Geometry: final body of the model. Coordinates: model frame, mm. A direction names the side the tool comes from. Give positions to 0.01 mm unless a question says otherwise; leave off trailing zeros. Write each loop counter-clockwise with the first axis right and the second up, starting at its lowest first coordinate (ties: lowest second). Pieces come first, ordered by that corner, then holes.
```python
from build123d import *

# Parameters (mm, degrees)
F0_W          = 19
F0_H          = 19
F3_DEPTH      = 2
F4_START      = 2
F2_W          = 19
F2_H          = 14
F4_DEPTH      = 9.5
F5_START      = 11.5
F1_R          = 6
F5_DEPTH      = 7.5
F6_R          = 1
F7_DEPTH      = 25
F7_DEPTH_BACK = 25
F8_R          = 5.2999998443
F9_DEPTH      = 1
F11_DEPTH     = 0.2
F12_R         = 0.5


# Not quite as in the source:
# - a fillet or chamfer that OpenCascade refuses, or shapes differently, is made with other operations: its cross-section is extruded or revolved along the edge and cut away or added


with BuildPart() as f3:
    # F0 (on Top) → F3 (new body)
    with BuildSketch(Plane.XY):
        Rectangle(F0_W, F0_H)
    extrude(amount=F3_DEPTH)

    # F2 (on Top) → F4 (join)
    with BuildSketch(Plane.XY.offset(F4_START)):
        Rectangle(F2_W, F2_H)
    extrude(amount=F4_DEPTH)

    # F1 (on Top) → F5 (join)
    with BuildSketch(Plane.XY.offset(F5_START)):
        Circle(F1_R)
    extrude(amount=F5_DEPTH)

    # F6 (on Right) → F7 (cut, two sides)
    with BuildSketch(Plane.YZ) as f7_sk:
        with Locations((0, 9)):
            Circle(F6_R)
    extrude(amount=-F7_DEPTH, mode=Mode.SUBTRACT)
    extrude(f7_sk.sketch, amount=F7_DEPTH_BACK, mode=Mode.SUBTRACT)

    # F8 (on face) → F9 (join)
    with BuildSketch(Plane.XY.offset(19)):
        Circle(F8_R)
    extrude(amount=F9_DEPTH)

    # F10: fillet of radius 14.5 on 1 edges, made by hand

    # F10_s1 → F10_t2 (revolve, cut)
    with BuildSketch(Plane.XZ):
        with BuildLine():
            ThreePointArc((5.2999998443, 19), (2.7010796257, 19.7478068488), (0.0084972222, 20))
            Line((0.0084972222, 20), (5.2999998443, 20))
            Line((5.2999998443, 20), (5.2999998443, 19))
        make_face()
    revolve(axis=Axis((0, 0, 20), (0, 0, 1)), mode=Mode.SUBTRACT)

    # F11 (add): a face of the model
    f11_faces = [f3.faces().sort_by_distance(p)[0] for p in [
        (-5.8302943725, 0, 19),
    ]]
    extrude(f11_faces, amount=F11_DEPTH)

    # F12
    f12_edges = [f3.edges().sort_by_distance(p)[0] for p in [
        (-6, 0, 19.2),
    ]]
    fillet(f12_edges, radius=F12_R)


solid = f3.part
```
Item 1: Reachability of faces 1 (the face through (0, -8, 2)), 2 (the face through (-0.1, 6.3, 11.5)), 3 (the face through (0, 8, 2)) from +Z, -Z, +X, -X, +Y, -Y: full face, straight path, thin tool, end or side. Return the list, or none.
Found:
face 1: +Z, +X, -X, -Y
face 2: +Z
face 3: +Z, +X, -X, +Y
Item 2: Section B-B, the plane z = 9. Return the cut outline in (x, y).
Found:
outline: (-9.5, -7) - (9.5, -7) - (9.5, -1) - (-9.5, -1) - close; (-9.5, 1) - (9.5, 1) - (9.5, 7) - (-9.5, 7) - close
Item 3: Pin query (flat end, axial travel): pin 1 Ø2 at (x, z) = (0.5, 6) entering from -Y; pin 2 Ø3 at (x, y) = (4.5, -8) entering from +Z; pin 3 Ø4 at (x, y) = (3.5, -2.5) entering from +Z. Return the tip coordinate at first contact, or that it passes through.
Found:
pin 1: stops at y = -7
pin 2: stops at z = 11.5
pin 3: stops at z = 19.82
Item 4: Section C-C, the plane y = -6.5. Return the cut outline in (x, z), plus the area to 4 significant figures.
Found:
outline: (-9.5, 0) - (9.5, 0) - (9.5, 11.5) - (-9.5, 11.5) - close
area: 218.5 mm2
Item 5: Pull-direction query (Y, two-part tool) for faces 4 (the face through (0, -9.5, 1)), 5 (the face through (0, 0, 0)), 6 (the face through (0, 0, 10)); classes: +Y half, -Y half, draft (parallel to the pull), parting line (faces both ways), or undercut.
Found:
face 4: -Y half
face 5: draft
face 6: undercut
Item 6: Section A-A, the plane x = 6.5. Return the cut outline in (y, z).
Found:
outline: (-9.5, 0) - (9.5, 0) - (9.5, 2) - (7, 2) - (7, 11.5) - (-7, 11.5) - (-7, 2) - (-9.5, 2) - close; hole circle Ø2 at (0, 9)
Item 7: Section D-D, the plane z = 16.25. Return the cut outline in (x, y).
Found:
outline: circle Ø12 at (0, 0)
Item 8: Line query: L1, parallel to Y at x = -3.75, z = 9; L2, parallel to Z at x = -5, y = -3.75; L3, parallel to Z at x = -3.5, y = 0.75. Output: solid intervals per line, ascending.
Found:
L1: y = -7 to -1, 1 to 7
L2: z = 0 to 11.5
L3: z = 0 to 8.34, 9.66 to 19.55
